Answer from the drawing. Dimensions are ordinates in mm from the lowest x, y and z of the part. A direction names the side the tool comes from. Coordinates: 2 decimals unless noted, no trailing zeros. Write each loop counter-clockwise with the first axis right and the second up, starting at its lowest first coordinate (ties: lowest second). Pieces come first, ordered by that corner, then holes.
(1) Which of the six approach directions +Z, -Z, +X, -X, +Y, -Y give full straight-line access (tool end or side, diameter ignored) to the marked faces 1, 2, 3, 4 and 5?
(2) The part is cut by section B-B on z = 48. Determine the outline of the cut face in (x, y) (1 decimal).
(3) Given P1, Ø4, axis at x = 48, y = 46.5, coming from the -Z side; P2, Ø7.5, axis at y = 50.5, z = 43.5, coming from the -X side, each flat-ended and moving along its own axis, determine where each tip first touches the part or whether it passes through.
(4) The part is cut by section C-C on x = 36.5. Determine the outline of the cut face in (y, z) (1 decimal), plus the area to 4 significant figures.
(5) Straight lines are drawn through the part: line 1 (Y direction, x = 6.5, z = 15.5) (1 decimal); line 2 (Y direction, x = 37, z = 41.5) (1 decimal); line 3 (X direction, y = 49.5, z = 72). For each, find the intervals that lie inside material, in ascending order.
(6) The part is cut by section A-A on x = 66.5. Determine the outline of the cut face in (y, z) (1 decimal).
(7) The part is cut by section D-D on y = 20. Determine the outline of the cut face in (x, z) (1 decimal), plus the area to 3 significant figures.
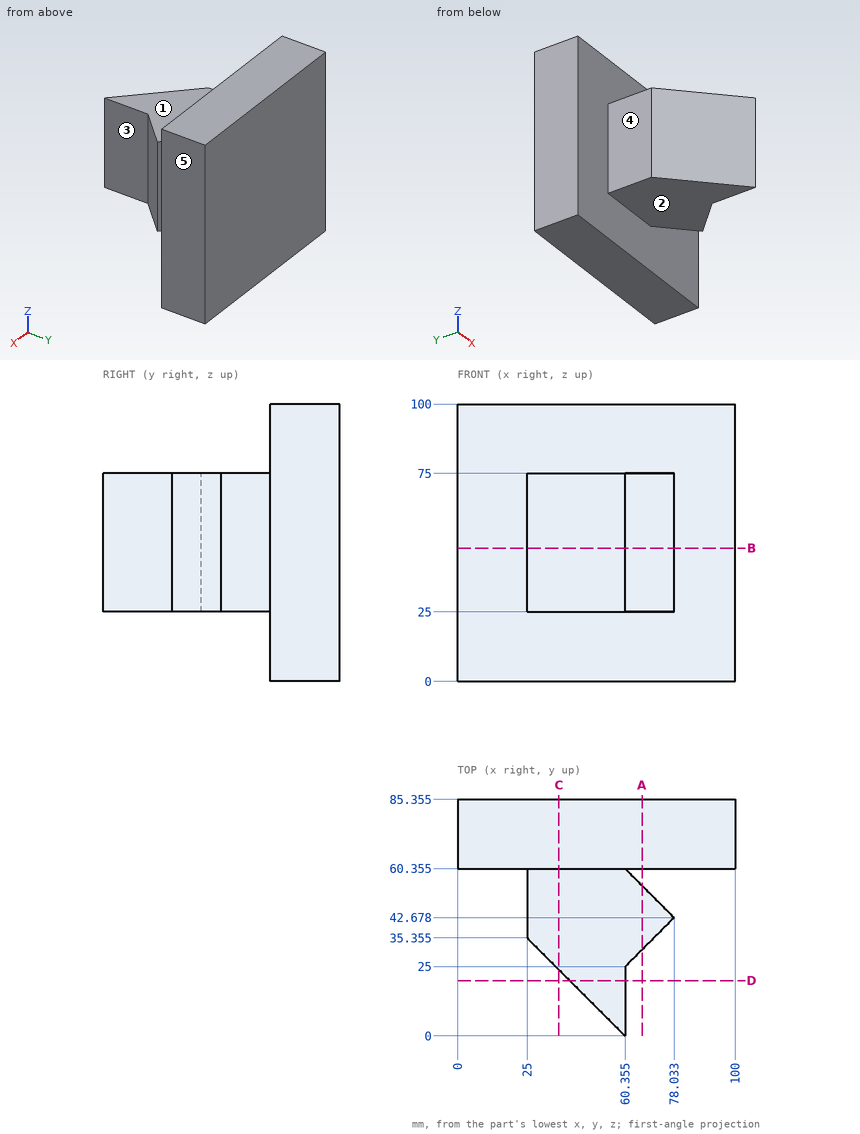
Model answer:
1. face 1: +Z, +X, -X, -Y
1. face 2: -Z, +X, -X, -Y
1. face 3: +Z, -Z, +X, -Y
1. face 4: +Z, -Z, -X, -Y
1. face 5: +Z, -Z, +X, +Y, -Y
2. outline: (0, 60.4) - (25, 60.4) - (25, 35.4) - (60.4, 0) - (60.4, 25) - (78, 42.7) - (60.4, 60.4) - (100, 60.4) - (100, 85.4) - (0, 85.4) - close
3. P1: stops at z = 25
3. P2: stops at x = 25
4. outline: (23.9, 25) - (60.4, 25) - (60.4, 0) - (85.4, 0) - (85.4, 100) - (60.4, 100) - (60.4, 75) - (23.9, 75) - close
4. area: 4,325 mm2
5. line 1: y = 60.4 to 85.4
5. line 2: y = 23.4 to 85.4
5. line 3: x = 25 to 71.21
6. outline: (31.1, 25) - (54.2, 25) - (54.2, 75) - (31.1, 75) - close; (60.4, 0) - (85.4, 0) - (85.4, 100) - (60.4, 100) - close
7. outline: (40.4, 25) - (60.4, 25) - (60.4, 75) - (40.4, 75) - close
7. area: 1,000 mm2
